Work out the finished part from the listing and answer in its coordinate system (mm). Face numbers are marked on the shaded views. A direction names the side the tool comes from. Round coordinates to 2 decimals unless told otherwise and drop trailing zeros. Order: outer loops, then holes, each group sorted by start corner. A loop starts at its lowest first (then second) coordinate and runs counter-clockwise, first axis right, second up.
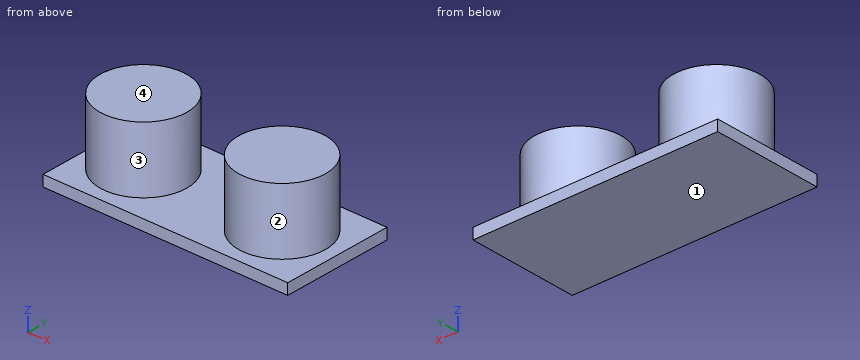
from build123d import *

# Parameters (mm, degrees)
SKETCH_1_W      = 45
SKETCH_1_H      = 20.5
EXTRUDE_1_DEPTH = 2
SKETCH_2_R      = 7.94
EXTRUDE_2_DEPTH = 12
SKETCH_3_R      = 7.94
EXTRUDE_3_DEPTH = 12


with BuildPart() as part:
    # 스케치1 → 보스-돌출1 (new body)
    with BuildSketch(Plane.XY):
        Rectangle(SKETCH_1_W, SKETCH_1_H)
    extrude(amount=EXTRUDE_1_DEPTH)

    # 스케치2 → 보스-돌출2 (add)
    with BuildSketch(Plane.XY.offset(2)):
        with Locations((-13.16, 0)):
            Circle(SKETCH_2_R)
    extrude(amount=EXTRUDE_2_DEPTH)

    # 스케치3 → 보스-돌출3 (add)
    with BuildSketch(Plane.XY.offset(2)):
        with Locations((12.34, 0)):
            Circle(SKETCH_3_R)
    extrude(amount=EXTRUDE_3_DEPTH)


solid = part.part
Item 1: A tool of negligible diameter and unlimited length cuts with its end or side. For the marked faces 3 and 4, from which of +Z, -Z, +X, -X, +Y, -Y can it reach the whole face along a straight path? Write none if from no direction.
Item 2: Find section A-A (y = 0). Write down the section's boundary in (x, z), plus the area to 3 significant figures.
Item 3: Find section C-C (x = 12.34). Write down the section's boundary in (y, z), plus the area to 3 significant figures.
Item 4: Find section D-D (y = -5.25). Write down the section's boundary in (x, z), plus the area to 3 significant figures.
Item 5: Find section B-B (z = 9.75). Write down the section's boundary in (x, y), plus the area to 3 significant figures.
Item 6: Given pin 1 (2 mm diameter, centred on y = -6, z = 8, fed in from -X); pin 2 (5 mm diameter, centred on y = 4.5, z = 7, fed in from +X); pin 3 (8 mm diameter, centred on x = 0.5, y = 4.5, fed in from +Z), each flat-ended and moving along its own axis, determine where each tip first touches the part or whether it passes through.
Item 7: For a pull along X with two mould halves and no side action, classify the marked faces 1 and 2 as released by +X, released by -X, zero draft, split by the parting line, or undercut.
Item 8: Find the intervals of material crossed by line 1 along Z through (x, y) = (6, -6.5); line 2 along X through (y, z) = (2.25, 10.25); line 3 along X through (y, z) = (6.75, 5.25), in increasing order.
Model answer:
1. face 3: +Z
1. face 4: +Z, +X, -X, +Y, -Y
2. outline: (-22.5, 0) - (22.5, 0) - (22.5, 2) - (20.28, 2) - (20.28, 14) - (4.4, 14) - (4.4, 2) - (-5.22, 2) - (-5.22, 14) - (-21.1, 14) - (-21.1, 2) - (-22.5, 2) - close
2. area: 471 mm2
3. outline: (-10.25, 0) - (10.25, 0) - (10.25, 2) - (7.94, 2) - (7.94, 14) - (-7.94, 14) - (-7.94, 2) - (-10.25, 2) - close
3. area: 232 mm2
4. outline: (-22.5, 0) - (22.5, 0) - (22.5, 2) - (18.3, 2) - (18.3, 14) - (6.38, 14) - (6.38, 2) - (-7.2, 2) - (-7.2, 14) - (-19.12, 14) - (-19.12, 2) - (-22.5, 2) - close
4. area: 376 mm2
5. outline: circle Ø15.88 at (-13.16, 0); circle Ø15.88 at (12.34, 0)
5. area: 396 mm2
6. pin 1: stops at x = -19.33
6. pin 2: stops at x = 20.02
6. pin 3: stops at z = 2
7. face 1: zero draft
7. face 2: undercut
8. line 1: z = 0 to 2
8. line 2: x = -20.77 to -5.55, 4.73 to 19.95
8. line 3: x = -17.34 to -8.98, 8.16 to 16.52
